from build123d import *

# Parameters (mm, degrees)
SKETCH1_R           = 1.98
SKETCH1_R_2         = 1.125
EXTRUDE1_DEPTH      = 522
SKETCH2_R           = 0.5
EXTRUDE2_DEPTH      = 2.98
EXTRUDE2_DEPTH_BACK = 2.98
SKETCH3_W           = 2.698417422
SKETCH3_H           = 6
EXTRUDE5_DEPTH      = 2


with BuildPart() as part:
    # Sketch1 → Extrude1 (new body)
    with BuildSketch(Plane.XY):
        Circle(SKETCH1_R)
        Circle(SKETCH1_R_2, mode=Mode.SUBTRACT)
    extrude(amount=EXTRUDE1_DEPTH)

    # Sketch2 → Extrude2 (cut, two sides)
    with BuildSketch(Plane(origin=(0, 0, 0), x_dir=(0, 0, -1), z_dir=(1, 0, 0))) as extrude2_sk:
        with Locations((-485, 1.5)):
            Circle(SKETCH2_R)
        with Locations((-17, 1.5)):
            Circle(SKETCH2_R)
    extrude(amount=EXTRUDE2_DEPTH, mode=Mode.SUBTRACT)
    extrude(extrude2_sk.sketch, amount=-EXTRUDE2_DEPTH_BACK, mode=Mode.SUBTRACT)

    # Sketch3 → Extrude5 (cut)
    with BuildSketch(Plane.XY):
        with Locations((1.849208711, 0)):
            Rectangle(SKETCH3_W, SKETCH3_H)
    extrude(amount=EXTRUDE5_DEPTH, mode=Mode.SUBTRACT)


solid = part.part
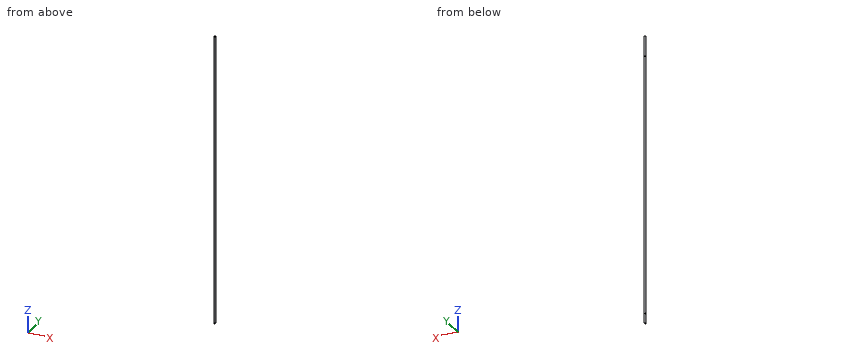
For this review, take the finished solid that the model builds, in its own axes (mm). Round coordinates to 2 decimals unless told otherwise and drop trailing zeros. Loops run counter-clockwise (first coordinate to the right, second up) from the corner with the lowest first, then second, coordinate; pieces in that order, holes last. Notation, with made-up numbers: (16.25, -27) - (37.25, -27) arc R22 cw to (37.25, -4) - close; hole circle Ø1 at (-9.5, 9.5). An arc over 180 degrees is marked (long way). One line per item, written item: value. Start each with the question number.
Item 1: Clearance check with flat-ended pins moving along their axes: pin 1 Ø0.5 at (y, z) = (1.5, 1) entering from +X; pin 2 Ø1.6 at (x, y) = (1, 0) entering from -Z. State where each tip first meets the part, or that it passes through.
Item 2: For L1, parallel to Z at x = -0.6, y = 1.5; L2, parallel to Z at x = 0.7, y = 1.5; L3, parallel to X at y = 0.1, z = 103, list the stretches that pass through material, from the lowest coordinate up.
Item 3: Take a section at B-B (z = 328). Give the boundary of the cut face in (x, y) (3 decimals), plus the area to 3 significant figures.
Item 4: Take a section at A-A (y = 0). Give the boundary of the cut face in (x, z) (3 decimals), plus the area to 3 significant figures.
Answer below:
1. pin 1: stops at x = 0.5
1. pin 2: stops at z = 2
2. L1: z = 0 to 16.5, 17.5 to 484.5, 485.5 to 522
2. L2: z = 2 to 16.5, 17.5 to 484.5, 485.5 to 522
2. L3: x = -1.98 to -1.12, 1.12 to 1.98
3. outline: circle Ø3.96 at (0, 0); hole circle Ø2.25 at (0, 0)
3. area: 8.34 mm2
4. outline: (-1.98, 0) - (-1.125, 0) - (-1.125, 522) - (-1.98, 522) - close; (1.125, 2) - (1.98, 2) - (1.98, 522) - (1.125, 522) - close
4. area: 891 mm2
